Source: CAD feature listing. Evaluate the final solid. Frame: model axes, mm. A direction names the side the tool comes from. Coordinates: 2 decimals unless noted, no trailing zeros. Order: outer loops, then holes, each group sorted by start corner. A loop starts at its lowest first (then second) coordinate and runs counter-clockwise, first axis right, second up. Notation, with made-up numbers: (67, 71) -> (117, 71) arc R31 cw to (117, 110) -> close; hole circle Ø1 at (59, 51). An arc over 180 degrees is marked (long way). Put each result on its own line as item: value.
from build123d import *

# Parameters (mm, degrees)
BOSS_EXTRUDE1_DEPTH              = 8
M30X2_0_TAPPED_HOLE5_D           = 28
M30X2_0_TAPPED_HOLE5_DEPTH       = 16
M30X2_0_TAPPED_HOLE5_CSINK_D     = 30.05
M30X2_0_TAPPED_HOLE5_CSINK_ANGLE = 90
M30X2_0_TAPPED_HOLE5_TIP         = 8.412048666


with BuildPart() as part:
    # Sketch1 → Boss-Extrude1 (new, symmetric)
    with BuildSketch(Plane(origin=(0, 0, 0), x_dir=(1, 0, 0), z_dir=(0, 1, 0))):
        with BuildLine():
            Line((4, -23.012812921), (4, -27.712812921))
            ThreePointArc((4, -27.712812921), (19.798989873, -19.798989873), (27.712812921, -4))
            Line((27.712812921, -4), (23.012812921, -4))
            Line((23.012812921, -4), (23.012812921, 4))
            Line((23.012812921, 4), (27.712812921, 4))
            ThreePointArc((27.712812921, 4), (19.798989873, 19.798989873), (4, 27.712812921))
            Line((4, 27.712812921), (4, 23.012812921))
            Line((4, 23.012812921), (-4, 23.012812921))
            Line((-4, 23.012812921), (-4, 27.712812921))
            ThreePointArc((-4, 27.712812921), (-19.798989873, 19.798989873), (-27.712812921, 4))
            Line((-27.712812921, 4), (-23.012812921, 4))
            Line((-23.012812921, 4), (-23.012812921, -4))
            Line((-23.012812921, -4), (-27.712812921, -4))
            ThreePointArc((-27.712812921, -4), (-19.798989873, -19.798989873), (-4, -27.712812921))
            Line((-4, -27.712812921), (-4, -23.012812921))
            Line((-4, -23.012812921), (4, -23.012812921))
        make_face()
    extrude(amount=BOSS_EXTRUDE1_DEPTH, both=True)

    # M30x2.0 Tapped Hole5
    with Locations(Plane(origin=(0, -8, 0), x_dir=(-1, 0, 0), z_dir=(0, -1, 0))):
        with Locations((0, 0)):
            CounterSinkHole(M30X2_0_TAPPED_HOLE5_D / 2, M30X2_0_TAPPED_HOLE5_CSINK_D / 2, depth=M30X2_0_TAPPED_HOLE5_DEPTH, counter_sink_angle=M30X2_0_TAPPED_HOLE5_CSINK_ANGLE)
            with Locations((0, 0, -(M30X2_0_TAPPED_HOLE5_DEPTH + M30X2_0_TAPPED_HOLE5_TIP / 2))):  # 118° drill point
                Cone(0, M30X2_0_TAPPED_HOLE5_D / 2, M30X2_0_TAPPED_HOLE5_TIP, mode=Mode.SUBTRACT)


solid = part.part
1. Cut plane D-D on x = 24.5. Output: boundary loops of the cut face in (y, z).
Numbers:
outline: (-8, -13.56) -> (8, -13.56) -> (8, -4) -> (-8, -4) -> close; (-8, 4) -> (8, 4) -> (8, 13.56) -> (-8, 13.56) -> close
2. Cut plane C-C on y = -2. Output: boundary loops of the cut face in (x, z), plus the area to 3 significant figures.
Numbers:
outline: (-27.71, -4) arc R28 ccw to (-4, -27.71) -> (-4, -23.01) -> (4, -23.01) -> (4, -27.71) arc R28 ccw to (27.71, -4) -> (23.01, -4) -> (23.01, 4) -> (27.71, 4) arc R28 ccw to (4, 27.71) -> (4, 23.01) -> (-4, 23.01) -> (-4, 27.71) arc R28 ccw to (-27.71, 4) -> (-23.01, 4) -> (-23.01, -4) -> close; hole circle Ø28 at (0, 0)
area: 1,690 mm2
3. First-contact query: pin 1 (4 mm diameter, centred on y = 2, z = 1.5, fed in from -X); pin 2 (1.4 mm diameter, centred on x = 26.5, y = 0.5, fed in from -Z); pin 3 (4 mm diameter, centred on x = -0.5, y = 1, fed in from -Z); pin 4 (9 mm diameter, centred on y = -3, z = -2, fed in from +X). Flat tips, straight axial feed; report the tip coordinate or a pass-through.
Numbers:
pin 1: stops at x = -23.01
pin 2: stops at z = -10.88
pin 3: stops at z = -23.01
pin 4: stops at x = 27.71
4. Pull-direction query (Z, two-part tool) for faces 1 (the flat face through (-25, 0, -4)), 2 (the flat face through (12, -8, 12)), 3 (the flat face through (0, 0, 23.013)); classes: pulls with the +Z half, pulls with the -Z half, needs draft (parallel to the pull), parting line crosses it, or undercut.
Numbers:
face 1: undercut
face 2: needs draft
face 3: pulls with the +Z half
5. Set-up query: faces 4 (the flat face through (25, 0, 4)), 5 (the flat face through (-23.013, 0, 0)), 6 (the flat face through (4, 0, 25)). Return all of +Z, -Z, +X, -X, +Y, -Y with unobstructed straight access to the full face (end or side cutting, diameter ignored); none if empty.
Numbers:
face 4: +X, +Y, -Y
face 5: -X, +Y, -Y
face 6: +Z, +Y, -Y
6. Ray query, line 1 along Z through (x, y) = (0, -3.25); line 2 along X through (y, z) = (2.5, 4.5); line 3 along X through (y, z) = (6, -13). Return the intervals inside material, ascending.
Numbers:
line 1: z = -23.01 to -14, 14 to 23.01
line 2: x = -27.64 to -13.26, 13.26 to 27.64
line 3: x = -24.8 to -5.2, 5.2 to 24.8
7. Cut plane A-A on z = 0. Output: boundary loops of the cut face in (x, y) (3 decimals).
Numbers:
outline: (-23.013, -8) -> (-15.025, -8) -> (-14, -6.975) -> (-14, 8) -> (-23.013, 8) -> close; (14, -6.975) -> (15.025, -8) -> (23.013, -8) -> (23.013, 8) -> (14, 8) -> close
8. Cut plane B-B on x = 0. Output: boundary loops of the cut face in (y, z) (3 decimals), plus the area to 3 significant figures.
Numbers:
outline: (-8, -23.013) -> (8, -23.013) -> (8, -14) -> (-6.975, -14) -> (-8, -15.025) -> close; (-8, 15.025) -> (-6.975, 14) -> (8, 14) -> (8, 23.013) -> (-8, 23.013) -> close
area: 287 mm2
